from build123d import *

# Parameters (mm, degrees)
SKETCH1_W               = 10
SKETCH1_H               = 10
SKETCH1_R               = 2.45
BASE_FLANGE1_DEPTH      = 1
EDGE_FLANGE1_DEPTH      = 10
EDGE_FLANGE1_BEND_DEPTH = 10
SKETCH12_R              = 2.45
CUT_EXTRUDE1_DEPTH      = 18.760630619
EDGE_FLANGE2_DEPTH      = 10
EDGE_FLANGE2_BEND_DEPTH = 10
SKETCH19_R              = 2.45
CUT_EXTRUDE2_DEPTH      = 21.385234351
CUT_EXTRUDE3_DEPTH      = 21.385234351


# Sheet-metal steps are written as plain solids
with BuildPart() as part:
    # Sketch1 → Base-Flange1 (new body)
    with BuildSketch(Plane(origin=(0, 0, 0), x_dir=(1, 0, 0), z_dir=(0, 1, 0))):
        Rectangle(SKETCH1_W, SKETCH1_H)
        with Locations(Location((0, 0, 0), (0, 0, 270))):
            Circle(SKETCH1_R, mode=Mode.SUBTRACT)
    extrude(amount=BASE_FLANGE1_DEPTH)

    # Edge-Flange1 section (across the edge) → Edge-Flange1 (add)
    with BuildSketch(Plane(origin=(-5.9, 1, -5), x_dir=(1, 0, 0), z_dir=(0, 0, 1))):
        with BuildLine():
            Line((-1, 0.9), (-1, 9))
            Line((-1, 9), (0, 9))
            Line((0, 9), (0, 0.9))
            ThreePointArc((0, 0.9), (0.263603897, 0.263603897), (0.9, 0))
            Line((0.9, 0), (0.9, -1))
            ThreePointArc((0.9, -1), (-0.443502884, -0.443502884), (-1, 0.9))
        make_face()
    extrude(amount=EDGE_FLANGE1_DEPTH)

    # Edge-Flange1 section 2 (across the edge) → Edge-Flange1 bend (add)
    with BuildSketch(Plane(origin=(5.9, 1, 5), x_dir=(-1, 0, 0), z_dir=(0, 0, -1))):
        with BuildLine():
            Line((-1, 0.9), (-1, 9))
            Line((-1, 9), (0, 9))
            Line((0, 9), (0, 0.9))
            ThreePointArc((0, 0.9), (0.263603897, 0.263603897), (0.9, 0))
            Line((0.9, 0), (0.9, -1))
            ThreePointArc((0.9, -1), (-0.443502884, -0.443502884), (-1, 0.9))
        make_face()
    extrude(amount=EDGE_FLANGE1_BEND_DEPTH)

    # Sketch12 → Cut-Extrude1 (cut, through all)
    with BuildSketch(Plane(origin=(6.9, 0, 0), x_dir=(0, 0, -1), z_dir=(1, 0, 0))):
        with Locations(Location((0, 5, 0), (0, 0, 90))):
            Circle(SKETCH12_R)
    extrude(amount=-CUT_EXTRUDE1_DEPTH, mode=Mode.SUBTRACT)

    # Edge-Flange2 section (across the edge) → Edge-Flange2 (add)
    with BuildSketch(Plane(origin=(6.9, 10.7366, -5), x_dir=(0, -1, 0), z_dir=(0, 0, 1))):
        with BuildLine():
            Line((-1, 0.7366), (-1, 9))
            Line((-1, 9), (0, 9))
            Line((0, 9), (0, 0.7366))
            ThreePointArc((0, 0.7366), (0.215745145, 0.215745145), (0.7366, 0))
            Line((0.7366, 0), (0.7366, -1))
            ThreePointArc((0.7366, -1), (-0.491361636, -0.491361636), (-1, 0.7366))
        make_face()
    extrude(amount=EDGE_FLANGE2_DEPTH)

    # Edge-Flange2 section 2 (across the edge) → Edge-Flange2 bend (add)
    with BuildSketch(Plane(origin=(-6.9, 10.7366, 5), x_dir=(0, -1, 0), z_dir=(0, 0, -1))):
        with BuildLine():
            Line((-1, 0.7366), (-1, 9))
            Line((-1, 9), (0, 9))
            Line((0, 9), (0, 0.7366))
            ThreePointArc((0, 0.7366), (0.215745145, 0.215745145), (0.7366, 0))
            Line((0.7366, 0), (0.7366, -1))
            ThreePointArc((0.7366, -1), (-0.491361636, -0.491361636), (-1, 0.7366))
        make_face()
    extrude(amount=EDGE_FLANGE2_BEND_DEPTH)

    # Sketch19 → Cut-Extrude2 (cut, through all)
    with BuildSketch(Plane(origin=(0, 11.7366, 0), x_dir=(1, 0, 0), z_dir=(0, 1, 0))):
        with Locations(Location((-10.9, 0, 0), (0, 0, 270))):
            Circle(SKETCH19_R)
        with Locations(Location((10.9, 0, 0), (0, 0, 270))):
            Circle(SKETCH19_R)
    extrude(amount=-CUT_EXTRUDE2_DEPTH, mode=Mode.SUBTRACT)

    # Sketch20 → Cut-Extrude3 (cut, through all)
    with BuildSketch(Plane(origin=(0, 11.7366, 0), x_dir=(1, 0, 0), z_dir=(0, 1, 0))):
        with BuildLine():
            Line((15.9, -5), (15.9, -3.1e-08))
            ThreePointArc((15.9, -3.1e-08), (14.435533895, -3.535533917), (10.9, -5))
            Line((10.9, -5), (15.9, -5))
        make_face()
        with BuildLine():
            Line((15.9, 5), (10.9, 5))
            ThreePointArc((10.9, 5), (14.435533917, 3.535533895), (15.9, -3.1e-08))
            Line((15.9, -3.1e-08), (15.9, 5))
        make_face()
        with BuildLine():
            ThreePointArc((-10.9, -5), (-14.435533906, -3.535533906), (-15.9, 0))
            Line((-15.9, 0), (-15.9, -5))
            Line((-15.9, -5), (-10.9, -5))
        make_face()
        with BuildLine():
            ThreePointArc((-15.9, 0), (-14.435533906, 3.535533906), (-10.9, 5))
            Line((-10.9, 5), (-15.9, 5))
            Line((-15.9, 5), (-15.9, 0))
        make_face()
    extrude(amount=-CUT_EXTRUDE3_DEPTH, mode=Mode.SUBTRACT)


solid = part.part
Design review of the part built by this model. Coordinates are the model's own, in mm. A direction names the side the tool comes from. Round coordinates to 2 decimals unless told otherwise and drop trailing zeros. Loops run counter-clockwise (first coordinate to the right, second up) from the corner with the lowest first, then second, coordinate; pieces in that order, holes last. Notation, with made-up numbers: (49.25, 73.25) -> (68.25, 73.25) arc R25 cw to (68.25, 93.25) -> close; hole circle Ø10 at (-25.5, 52). An arc over 180 degrees is marked (long way). Use one line per item in the form item = value. Start each with the question number.
Q1. Machinability: for faces 1 (the face through (-14, 11.737, 0)), 2 (the face through (-14, 10.737, 0)), 3 (the face through (14, 10.737, 0)), 4 (the face through (6.395, 11.214, -0.07)), which of the approach directions +Z, -Z, +X, -X, +Y, -Y give a long, thin tool a straight path to every point of the face, cutting with its end or side? Answer none if there is none.
Q2. Draft analysis for pull direction X (two halves, no side actions). For faces 5 (the face through (6.407, 7.263, -0.938)), 6 (the face through (-5.9, 8, 0)), 7 (the face through (-6.9, 8, 0)), state which applies: +X half, -X half, draft (parallel to the pull), parting line (faces both ways), or undercut.
Q3. We need section A-A on y = 8.25. Give the boundary of the cut face in (x, z).
Q4. We need section B-B on x = 0. Give the boundary of the cut face in (y, z), then the cut area to 3 significant figures.
Q5. For pin 1 Ø1 at (x, y) = (-5, 3) entering from -Z; pin 2 Ø3 at (y, z) = (4.5, -3) entering from +X; pin 3 Ø5 at (x, z) = (2.5, 0) entering from +Y, all flat-tipped, find the tip position at first contact; note any pin that passes through.
Q6. Wall thickness on line 1 along X through (y, z) = (7.25, -2); line 2 along Y through (x, z) = (-0.5, 3.25); line 3 along Y through (x, z) = (-14, -2.25): over which ranges is each line inside the solid? List them lowest first. Write a range as [from, to].
Q7. We need section D-D on z = -3.5. Give the boundary of the cut face in (x, y).
Q8. We need section C-C on y = 5. Give the boundary of the cut face in (x, z).
Calculated:
q1.face_1 = +Z, -Z, +X, -X, +Y
q1.face_2 = +Z, -Z, -X, -Y
q1.face_3 = +Z, -Z, +X, -Y
q1.face_4 = +Z, -Z, +Y
q2.face_5 = draft
q2.face_6 = undercut
q2.face_7 = -X half
q3.outline = (-6.9, -5) -> (-5.9, -5) -> (-5.9, 5) -> (-6.9, 5) -> close; (5.9, -5) -> (6.9, -5) -> (6.9, 5) -> (5.9, 5) -> close
q4.outline = (0, -5) -> (1, -5) -> (1, -2.45) -> (0, -2.45) -> close; (0, 2.45) -> (1, 2.45) -> (1, 5) -> (0, 5) -> close
q4.area = 5.10 mm²
q5.pin_1 = through
q5.pin_2 = 6.9
q5.pin_3 = 1
q6.line_1 = [-6.9, -5.9], [5.9, 6.9]
q6.line_2 = [0, 1]
q6.line_3 = [10.74, 11.74]
q7.outline = (-14.47, 10.74) -> (-7.64, 10.74) arc R0.74 cw to (-6.9, 10) -> (-6.9, 1.9) arc R1.9 ccw to (-5, 0) -> (5, 0) arc R1.9 ccw to (6.9, 1.9) -> (6.9, 10) arc R0.74 cw to (7.64, 10.74) -> (14.47, 10.74) -> (14.47, 11.74) -> (7.64, 11.74) arc R1.74 ccw to (5.9, 10) -> (5.9, 1.9) arc R0.9 cw to (5, 1) -> (-5, 1) arc R0.9 cw to (-5.9, 1.9) -> (-5.9, 10) arc R1.74 ccw to (-7.64, 11.74) -> (-14.47, 11.74) -> close
q8.outline = (-6.9, -5) -> (-5.9, -5) -> (-5.9, -2.45) -> (-6.9, -2.45) -> close; (-6.9, 2.45) -> (-5.9, 2.45) -> (-5.9, 5) -> (-6.9, 5) -> close; (5.9, -5) -> (6.9, -5) -> (6.9, -2.45) -> (5.9, -2.45) -> close; (5.9, 2.45) -> (6.9, 2.45) -> (6.9, 5) -> (5.9, 5) -> close
